Verification items for the finished model (mm, model axes). Face numbers are marked on the shaded views. Coordinates: 2 decimals unless noted, no trailing zeros. Write each loop counter-clockwise with the first axis right and the second up, starting at its lowest first coordinate (ties: lowest second). Pieces come first, ordered by that corner, then holes. Notation, with made-up numbers: M 48.5,21.25 L 67.5,21.25 A9 ccw 67.5,27.25 Z; hole C 79,40 d10. An arc over 180 degrees is marked long. Answer in a Markdown table with one row per item.
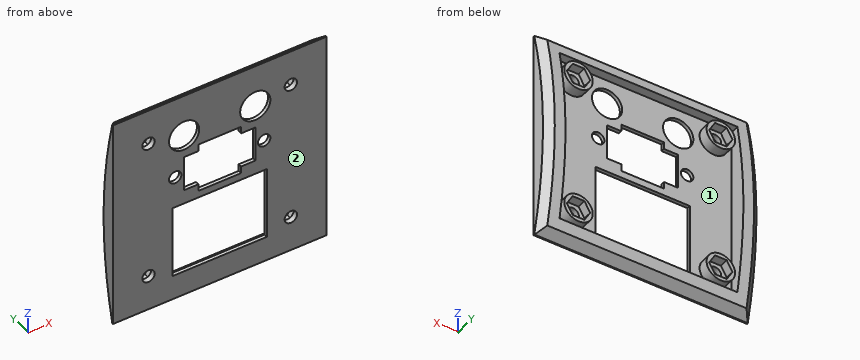
Autodesk Inventor part; units mm, degrees
ref_plane "Work Plane1" through (30, 6, 0) normal (0, -1, 0) x (1, 0, 0)
ref_plane "YZ Plane" through (0, 0, 0) normal (1, 0, 0) x (0, 1, 0)
ref_plane "XZ Plane" through (0, 0, 0) normal (0, 1, 0) x (-1, 0, 0)
sketch "Sketch1" plane through (0, 0, 0) normal (0, 1, 0) x (-1, 0, 0)
  line L0 (30, 30) -> (-30, 30)
  line L1 (-30, 30) -> (-30, -30)
  line L2 (-30, -30) -> (30, -30)
  line L3 (30, -30) -> (30, 30)
  line L4 (30, 30) -> (-30, -30) construction
  line L5 (-30, 30) -> (30, -30) construction
  point P0 (0, 0)
  dimension "d0" = 60
  dimension "d1" = 60
extrude "Extrusion1" add sketch "Sketch1" along normal blind 6
sketch "Sketch2" plane through (30, 0, 30) normal (1, 0, 0) x (0, 0, -1)
  circle A0 centre (30, -119) radius 125
  line L0 (0, 6) -> (60, 6)
  line L1 (0, 0) -> (60, 0)
  point P0 (30, 0)
  point P1 (30, 0)
  dimension "d4" = 250
extrude "Extrusion2" cut sketch "Sketch2" against normal through all keep common part
ref_plane "Work Plane1" through (30, 6, 0) normal (0, -1, 0) x (1, 0, 0)
sketch "Sketch3" plane through (30, 6, 0) normal (0, -1, 0) x (1, 0, 0)
  line L0 (-55, -25) -> (-5, -25)
  line L1 (-5, -25) -> (-5, 25)
  line L2 (-5, 25) -> (-55, 25)
  line L3 (-55, 25) -> (-55, -25)
  line L4 (-55, -25) -> (-5, 25) construction
  line L5 (-5, -25) -> (-55, 25) construction
  line L6 (0, -30) -> (-60, -30)
  line L7 (0, 30) -> (0, -30)
  point P0 (-30, 0)
  point P1 (-30, 0)
  dimension "d19" = 5
  dimension "d20" = 5
extrude "Extrusion3" cut sketch "Sketch3" along normal blind 5
sketch "Sketch4" plane through (30, 1, 0) normal (0, 1, 0) x (1, 0, 0)
  line L0 (-43.25, 23) -> (-16.75, 23)
  line L1 (-16.75, 23) -> (-16.75, 2.5)
  line L2 (-16.75, 2.5) -> (-43.25, 2.5)
  line L3 (-43.25, 2.5) -> (-43.25, 23)
  line L4 (-43.25, 23) -> (-16.75, 2.5) construction
  line L5 (-16.75, 23) -> (-43.25, 2.5) construction
  line L6 (-55, 25) -> (-5, 25)
  line L7 (-30, 12.75) -> (-30, 10.9588)
  line L8 (-40, -1.5) -> (-20, -1.5)
  line L9 (-20, -1.5) -> (-20, -11.5)
  line L10 (-20, -11.5) -> (-40, -11.5)
  line L11 (-40, -11.5) -> (-40, -1.5)
  line L12 (-40, -1.5) -> (-20, -11.5) construction
  line L13 (-20, -1.5) -> (-40, -11.5) construction
  circle A0 centre (-42.5, -6.5) radius 1.75
  circle A1 centre (-17.5, -6.5) radius 1.75
  circle A2 centre (-40, -18) radius 4.25
  circle A3 centre (-20, -18) radius 4.25
  line L14 (-24, -13.5) -> (-36, -13.5)
  line L15 (-36, -13.5) -> (-36, -11.5)
  line L16 (-36, -11.5) -> (-24, -11.5)
  line L17 (-24, -11.5) -> (-24, -13.5)
  line L18 (-24, -13.5) -> (-36, -11.5) construction
  line L19 (-36, -13.5) -> (-24, -11.5) construction
  line L20 (-24, 0.5) -> (-36, 0.5)
  line L21 (-36, 0.5) -> (-36, -1.5)
  line L22 (-36, -1.5) -> (-24, -1.5)
  line L23 (-24, -1.5) -> (-24, 0.5)
  line L24 (-24, 0.5) -> (-36, -1.5) construction
  line L25 (-36, 0.5) -> (-24, -1.5) construction
  line L26 (0, 30) -> (-60, 30)
  point P0 (-30, 0)
  point P1 (-30, -6.5)
  point P2 (-30, -12.5)
  point P3 (-30, -0.5)
  point P4 (-24, -11.5)
  point P5 (-24, -1.5)
  dimension "d11" = 20.5
  dimension "d12" = 26.5
  dimension "d13" = 2
  dimension "d26" = 10
  dimension "d27" = 20
  dimension "d28" = 4
  dimension "d29" = 3.5
  dimension "d30" = 3.5
  dimension "d31" = 25
  dimension "d38" = 8.5
  dimension "d42" = 20
  dimension "d43" = 12
  dimension "d44" = 2
  dimension "d45" = 12
  dimension "d46" = 2
  dimension "d64" = 48
extrude "Extrusion4" cut sketch "Sketch4" against normal through all contours L0 L1 L2 L3
chamfer "Chamfer1" distance 2 angle 45 4 edges at (-30, 6, 0) (0, 2.3466, -30) (30, 6, 0) (0, 2.3466, 30)
extrude "Extrusion6" cut sketch "Sketch4" against normal blind 10 contours L8 L9 L10 L11 | L21 L20 L23 L8 | L10 L17 L14 L15
extrude "Extrusion7" cut sketch "Sketch4" against normal through all contours A0 | A1
sketch "Sketch8" plane through (30, 1, 0) normal (0, 1, 0) x (1, 0, 0)
  line L0 (-30, -21.9563) -> (-30, 0)
  line L1 (-30, 0) -> (-52.0851, 0)
  line L2 (-24, 0.5) -> (-36, 0.5)
  circle A0 centre (-10, -20) radius 4
  circle A1 centre (-50, -20) radius 4
  circle A2 centre (-10, 20) radius 4
  circle A3 centre (-50, 20) radius 4
  dimension "d56" = 8
  dimension "d57" = 40
  dimension "d58" = 40
extrude "Extrusion11" add sketch "Sketch8" along normal blind 3
sketch "Sketch9" plane through (20, 4, 20) normal (0, 1, 0) x (1, 0, 0)
  circle A0 centre (0, 0) radius 4
  line L0 (-3.2909, 0) -> (-1.6454, 2.85)
  line L1 (-1.6454, 2.85) -> (1.6454, 2.85)
  line L2 (1.6454, 2.85) -> (3.2909, 0)
  line L3 (3.2909, 0) -> (1.6454, -2.85)
  line L4 (1.6454, -2.85) -> (-1.6454, -2.85)
  line L5 (-1.6454, -2.85) -> (-3.2909, 0)
  line L6 (-20, 20) -> (-20, -14.7527)
  line L7 (-20, 20) -> (-56.1519, 20)
  line L8 (-36.7091, 0) -> (-38.3546, 2.85)
  line L9 (-38.3546, 2.85) -> (-41.6454, 2.85)
  line L10 (-41.6454, 2.85) -> (-43.2909, 0)
  line L11 (-43.2909, 0) -> (-41.6454, -2.85)
  line L12 (-41.6454, -2.85) -> (-38.3546, -2.85)
  line L13 (-38.3546, -2.85) -> (-36.7091, 0)
  line L14 (-3.2909, 40) -> (-1.6454, 37.15)
  line L15 (-1.6454, 37.15) -> (1.6454, 37.15)
  line L16 (1.6454, 37.15) -> (3.2909, 40)
  line L17 (3.2909, 40) -> (1.6454, 42.85)
  line L18 (1.6454, 42.85) -> (-1.6454, 42.85)
  line L19 (-1.6454, 42.85) -> (-3.2909, 40)
  line L20 (-43.2909, 40) -> (-41.6454, 42.85)
  line L21 (-41.6454, 42.85) -> (-38.3546, 42.85)
  line L22 (-38.3546, 42.85) -> (-36.7091, 40)
  line L23 (-36.7091, 40) -> (-38.3546, 37.15)
  line L24 (-38.3546, 37.15) -> (-41.6454, 37.15)
  line L25 (-41.6454, 37.15) -> (-43.2909, 40)
  dimension "d61" = 5.7
extrude "Extrusion12" cut sketch "Sketch9" against normal blind 2.5 contours L0 L1 L2 L3 L4 L5 | L13 L12 L11 L10 L9 L8 | L19 L18 L17 L16 L15 L14 | L20 L21 L22 L23 L24 L25
extrude "Extrusion9" cut sketch "Sketch4" against normal through all contours A2 | A3
sketch "Sketch11" plane through (20, 1.5, 20) normal (0, 1, 0) x (1, 0, 0)
  circle A0 centre (0, 0) radius 1.75
  circle A1 centre (-40, 0) radius 1.75
  circle A2 centre (-40, 40) radius 1.75
  circle A3 centre (0, 40) radius 1.75
  point P0 (-20, 20)
  dimension "d72" = 3.5
  dimension "d73" = 3.5
  dimension "d74" = 3.5
  dimension "d75" = 3.5
extrude "Extrusion13" cut sketch "Sketch11" against normal through all
sketch "Sketch7" plane through (30, 1, 0) normal (0, 1, 0) x (1, 0, 0)
  circle A0 centre (-10, -6.5) radius 1.65
  circle A1 centre (-50, -6.5) radius 1.65
  line L0 (-30, -18.5284) -> (-30, 12.7052) construction
  circle A2 centre (-17.5, -6.5) radius 1.75 construction
  point P0 (-30, 0)
  dimension "d52" = 3.3
  dimension "d53" = 40
equation "\"d30\" = d29"
equation "\"d45\" = d43"
equation "\"d46\" = d44"
equation "\"d73\" = d72"
equation "\"d74\" = d72"
equation "\"d75\" = d72"
properties part number "power_signal_socket" material "Acetal Resin, Black"
1) Thickness scan on L1, parallel to X at y = 0.55, z = 6.5; L2, parallel to X at y = 0.5, z = -8.5; L3, parallel to X at y = 0.6, z = -20. Record the ranges inside material, lowest first. Write a range as [from, to].
Response values:
| item | result |
|---|---|
| L1 | x = [-30, -14.25], [-10.75, -10], [10, 10.75], [14.25, 30] |
| L2 | x = [-30, -13.25], [13.25, 30] |
| L3 | x = [-30, -21.75], [-18.25, -13.25], [13.25, 18.25], [21.75, 30] |
2) Sectioned sample at A-A (x = -20). Give the number of separate pieces and of enclosed holes in the cut face, then the cut area to 3 significant figures.
Response values:
| item | result |
|---|---|
| separate pieces | 3 |
| enclosed holes | 0 |
| area | 84.4 mm² |
3) Depth check by flat-ended pin: pin 1 (6.5 mm diameter, centred on x = -21, z = 20, fed in from +Y); pin 2 (2 mm diameter, centred on x = -1.5, y = 2, fed in from -Z); pin 3 (1.2 mm diameter, centred on x = 20.5, y = 2.5, fed in from -Z). Enter the tip coordinate at first touch or a pass-through.
Response values:
| item | result |
|---|---|
| pin 1 | stops at y = 4 |
| pin 2 | stops at z = -29.48 |
| pin 3 | stops at z = -28.77 |
4) Sectioned sample at B-B (x = -7). Record the cut outline in (y, z), then the cut area to 3 significant figures.
Response values:
| item | result |
|---|---|
| outline | M 0,-30 L 0.35,-30 L 2.81,-28.05 A125 ccw 3.47,-25 L 1,-25 L 1,-23 L 0,-23 Z; M 0,-2.5 L 1,-2.5 L 1,1.5 L 0,1.5 Z; M 0,11.5 L 1,11.5 L 1,14.99 L 0,14.99 Z; M 0,21.01 L 1,21.01 L 1,25 L 3.47,25 A125 ccw 2.81,28.05 L 0.35,30 L 0,30 Z |
| area | 38.9 mm² |
5) Release check for a two-part mould opening along X. For the marked faces 1 and 2 record: +X half, -X half, draft (parallel to the pull), parting line (faces both ways), or undercut.
Response values:
| item | result |
|---|---|
| face 1 | undercut |
| face 2 | draft |
